```python
from build123d import *

# Parameters (mm, degrees)
F0_R     = 3.5
F1_DEPTH = 3.5


with BuildPart() as f1:
    # F0 (on Top) → F1 (new body)
    with BuildSketch(Plane.XY):
        with BuildLine():
            Line((17.412545, 2.5), (20.258875, 2.5))
            ThreePointArc((20.258875, 2.5), (0, 20.412545), (-20.258875, 2.5))
            Line((-20.258875, 2.5), (-17.412545, 2.5))
            Line((-17.412545, 2.5), (-17.412545, -2.5))
            Line((-17.412545, -2.5), (-20.258875, -2.5))
            ThreePointArc((-20.258875, -2.5), (-19.203199, -6.921644), (-17.195116, -11))
            Line((-17.195116, -11), (-12, -11))
            ThreePointArc((-12, -11), (-9, -8), (-6, -11))
            Line((-6, -11), (-3, -11))
            ThreePointArc((-3, -11), (0, -8), (3, -11))
            Line((3, -11), (6, -11))
            ThreePointArc((6, -11), (9, -8), (12, -11))
            Line((12, -11), (17.195116, -11))
            ThreePointArc((17.195116, -11), (19.203199, -6.921644), (20.258875, -2.5))
            Line((20.258875, -2.5), (17.412545, -2.5))
            Line((17.412545, -2.5), (17.412545, 2.5))
        make_face()
        Circle(F0_R, mode=Mode.SUBTRACT)
        with BuildLine():
            ThreePointArc((-17.195116, -11), (0, -20.412545), (17.195116, -11))
            Line((17.195116, -11), (12, -11))
            ThreePointArc((12, -11), (9, -14), (6, -11))
            Line((6, -11), (3, -11))
            ThreePointArc((3, -11), (0, -14), (-3, -11))
            Line((-3, -11), (-6, -11))
            ThreePointArc((-6, -11), (-9, -14), (-12, -11))
            Line((-12, -11), (-17.195116, -11))
        make_face()
        with BuildLine():
            Line((-17.412545, 2.5), (-20.258875, 2.5))
            ThreePointArc((-20.258875, 2.5), (-20.412545, 0), (-20.258875, -2.5))
            Line((-20.258875, -2.5), (-17.412545, -2.5))
            Line((-17.412545, -2.5), (-17.412545, 2.5))
        make_face()
        with BuildLine():
            ThreePointArc((-20.258875, -2.5), (-20.412545, 0), (-20.258875, 2.5))
            Line((-20.258875, 2.5), (-23.412545, 2.5))
            Line((-23.412545, 2.5), (-23.412545, -2.5))
            Line((-23.412545, -2.5), (-20.258875, -2.5))
        make_face()
        with BuildLine():
            ThreePointArc((20.258875, -2.5), (20.374091, -1.252359), (20.412545, 0))
            ThreePointArc((20.412545, 0), (20.374091, 1.252359), (20.258875, 2.5))
            Line((20.258875, 2.5), (17.412545, 2.5))
            Line((17.412545, 2.5), (17.412545, -2.5))
            Line((17.412545, -2.5), (20.258875, -2.5))
        make_face()
        with BuildLine():
            ThreePointArc((20.258875, 2.5), (20.374091, 1.252359), (20.412545, 0))
            ThreePointArc((20.412545, 0), (20.374091, -1.252359), (20.258875, -2.5))
            Line((20.258875, -2.5), (23.412545, -2.5))
            Line((23.412545, -2.5), (23.412545, 2.5))
            Line((23.412545, 2.5), (20.258875, 2.5))
        make_face()
    extrude(amount=F1_DEPTH)


solid = f1.part
```
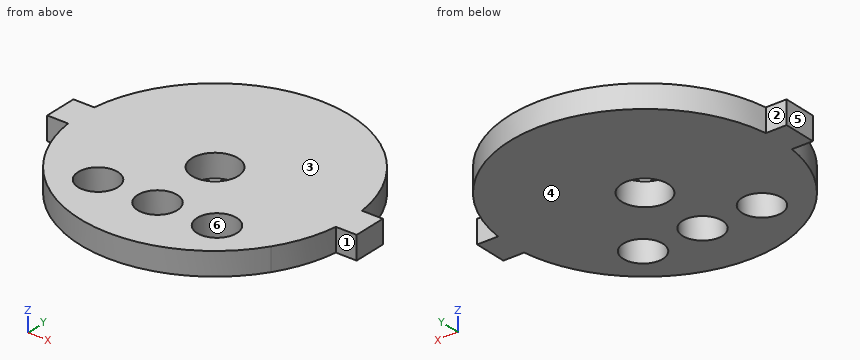
Input: part model. Units: mm. Frame: model coordinates. Face numbers are marked on the shaded views. A direction names the side the tool comes from. Round coordinates to 2 decimals unless told otherwise and drop trailing zeros. Write each loop counter-clockwise with the first axis right and the second up, starting at its lowest first coordinate (ties: lowest second). Pieces come first, ordered by that corner, then holes. Notation, with made-up numbers: (79.25, 17.5) -> (98.25, 17.5) arc R14 cw to (98.25, 30.5) -> close; hole circle Ø8 at (86, -30.5). An arc over 180 degrees is marked (long way). Answer as CSV lines item,"result".
1. Section D-D (y = -8.5). Return the cut outline in (x, z), plus the area to 3 significant figures.
Geometry says:
outline,"(-18.56, 0) -> (-10.66, 0) -> (-10.66, 3.5) -> (-18.56, 3.5) -> close; (-7.34, 0) -> (-1.66, 0) -> (-1.66, 3.5) -> (-7.34, 3.5) -> close; (1.66, 0) -> (7.34, 0) -> (7.34, 3.5) -> (1.66, 3.5) -> close; (10.66, 0) -> (18.56, 0) -> (18.56, 3.5) -> (10.66, 3.5) -> close"
area,"95.1 mm^2"
2. Section B-B (y = 0). Return the cut outline in (x, z).
Geometry says:
outline,"(-23.41, 0) -> (-3.5, 0) -> (-3.5, 3.5) -> (-23.41, 3.5) -> close; (3.5, 0) -> (23.41, 0) -> (23.41, 3.5) -> (3.5, 3.5) -> close"
3. Mould query, pull axis X, two halves, no side actions, for the marked faces 4, 5 and 6. Classes: +X half, -X half, draft (parallel to the pull), parting line (faces both ways), or undercut.
Geometry says:
face 4,"draft"
face 5,"-X half"
face 6,"undercut"
4. Ray query, L1, parallel to X at y = -11, z = 2.6; L2, parallel to Y at x = 0, z = 2; L3, parallel to Y at x = -20.5, z = 0.95. Return the intervals inside material, ascending. Write a range as [from, to].
Geometry says:
L1,"x = [-17.2, -12], [-6, -3], [3, 6], [12, 17.2]"
L2,"y = [-20.41, -14], [-8, -3.5], [3.5, 20.41]"
L3,"y = [-2.5, 2.5]"
5. Section A-A (x = 0). Return the cut outline in (y, z), plus the area to 3 significant figures.
Geometry says:
outline,"(-20.41, 0) -> (-14, 0) -> (-14, 3.5) -> (-20.41, 3.5) -> close; (-8, 0) -> (-3.5, 0) -> (-3.5, 3.5) -> (-8, 3.5) -> close; (3.5, 0) -> (20.41, 0) -> (20.41, 3.5) -> (3.5, 3.5) -> close"
area,"97.4 mm^2"
6. Reachability of the marked faces 1, 2 and 3 from +Z, -Z, +X, -X, +Y, -Y: full face, straight path, thin tool, end or side. Return the list, or none.
Geometry says:
face 1,"+Z, -Z, +X, -Y"
face 2,"+Z, -Z, -X, +Y"
face 3,"+Z, +X, -X, +Y, -Y"
7. Section C-C (z = 1.95). Return the cut outline in (x, y), plus the area to 3 significant figures.
Geometry says:
outline,"(-23.41, -2.5) -> (-20.26, -2.5) arc R20.41 ccw to (-17.2, -11) arc R20.41 ccw to (17.2, -11) arc R20.41 ccw to (20.26, -2.5) -> (23.41, -2.5) -> (23.41, 2.5) -> (20.26, 2.5) arc R20.41 ccw to (-20.26, 2.5) -> (-23.41, 2.5) -> close; hole circle Ø6 at (-9, -11); hole circle Ø7 at (0, 0); hole circle Ø6 at (0, -11); hole circle Ø6 at (9, -11)"
area,"1,220 mm^2"
